Read the model definition and answer for the solid it produces. Units are mm, in the model's axes. Coordinates: 2 decimals unless noted, no trailing zeros. Loops run counter-clockwise (first coordinate to the right, second up) from the corner with the lowest first, then second, coordinate; pieces in that order, holes last. Notation, with made-up numbers: (86.5, 80.5) - (113.5, 80.5) arc R23 ccw to (113.5, 112.5) - close; hole circle Ø3 at (13.5, 31.5). An arc over 180 degrees is marked (long way). One line per item, written item: value. Start each with the question number.
from build123d import *

# Parameters (mm, degrees)
F0_W     = 35
F0_H     = 22
F0_R     = 3.5
F1_DEPTH = 1.3
F2_R     = 6
F3_R     = 0.5


with BuildPart() as f1:
    # F0 (on Top) → F1 (new body)
    with BuildSketch(Plane.XY):
        with Locations((0, 2.5)):
            Rectangle(F0_W, F0_H)
        Circle(F0_R, mode=Mode.SUBTRACT)
    extrude(amount=F1_DEPTH)

    # F2
    f2_edges = [f1.edges().sort_by_distance(p)[0] for p in [
        (17.5, 13.5, 0.65),
        (-17.5, 13.5, 0.65),
        (-17.5, -8.5, 0.65),
        (17.5, -8.5, 0.65),
    ]]
    fillet(f2_edges, radius=F2_R)

    # F3
    f3_edges = [f1.edges().sort_by_distance(p)[0] for p in [
        (0, 13.5, 1.3),
        (15.742641, 11.742641, 1.3),
        (-15.742641, 11.742641, 1.3),
        (17.5, 2.5, 1.3),
        (-17.5, 2.5, 1.3),
        (15.742641, -6.742641, 1.3),
        (-15.742641, -6.742641, 1.3),
        (0, -8.5, 1.3),
        (-3.5, 0, 1.3),
    ]]
    fillet(f3_edges, radius=F3_R)


solid = f1.part
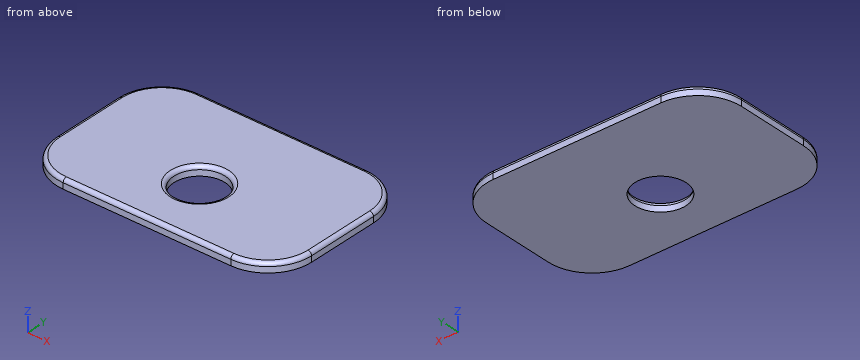
1) Straight lines are drawn through the part: L1, parallel to Y at x = 0, z = 0.2; L2, parallel to X at y = -1.25, z = 0.8; L3, parallel to Y at x = -15, z = 0.55. For each, find the intervals that lie inside material, in ascending order.
2) Section C-C, the plane z = 0.55 is taken. Determine the outline of the cut face in (x, y).
3) Section B-B, the plane y = 0 is taken. Determine the outline of the cut face in (x, z), and give its area (3 significant figures).
4) Section A-A, the plane x = 0 is taken. Determine the outline of the cut face in (y, z).
Answer below:
1. L1: -8.5 to -3.5, 3.5 to 13.5
1. L2: -17.5 to -3.27, 3.27 to 17.5
1. L3: -7.37 to 12.37
2. outline: (-17.5, -2.5) arc R6 ccw to (-11.5, -8.5) - (11.5, -8.5) arc R6 ccw to (17.5, -2.5) - (17.5, 7.5) arc R6 ccw to (11.5, 13.5) - (-11.5, 13.5) arc R6 ccw to (-17.5, 7.5) - close; hole circle Ø7 at (0, 0)
3. outline: (-17.5, 0) - (-3.5, 0) - (-3.5, 0.8) arc R0.5 ccw to (-4, 1.3) - (-17, 1.3) arc R0.5 ccw to (-17.5, 0.8) - close; (3.5, 0) - (17.5, 0) - (17.5, 0.8) arc R0.5 ccw to (17, 1.3) - (4, 1.3) arc R0.5 ccw to (3.5, 0.8) - close
3. area: 36.2 mm2
4. outline: (-8.5, 0) - (-3.5, 0) - (-3.5, 0.8) arc R0.5 ccw to (-4, 1.3) - (-8, 1.3) arc R0.5 ccw to (-8.5, 0.8) - close; (3.5, 0) - (13.5, 0) - (13.5, 0.8) arc R0.5 ccw to (13, 1.3) - (4, 1.3) arc R0.5 ccw to (3.5, 0.8) - close
